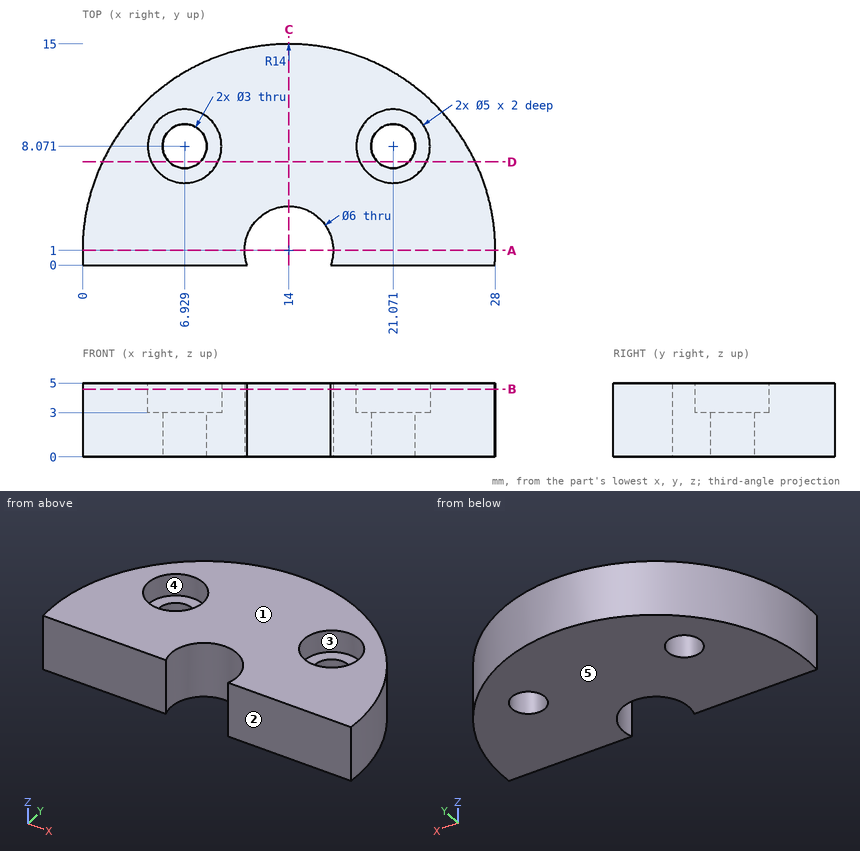
Check sheet for the drawn part. Datum: minimum x, y, z corner. Units: mm. A direction names the side the tool comes from. Round coordinates to 2 decimals unless told otherwise and drop trailing zeros. Loops run counter-clockwise (first coordinate to the right, second up) from the corner with the lowest first, then second, coordinate; pieces in that order, holes last. Notation, with made-up numbers: (-37, 59.25) - (-15, 59.25) arc R28 cw to (-15, 98.25) - close; hole circle Ø3 at (89.5, 28.25). An arc over 180 degrees is marked (long way). Write item = value, one per line. Start each with the question number.
1. Depth check by flat-ended pin: pin 1 (7 mm diameter, centred on x = 14, y = 1, fed in from +Z); pin 2 (1 mm diameter, centred on y = 12, z = 4, fed in from +X); pin 3 (2 mm diameter, centred on x = 13.5, z = 2, fed in from -Y); pin 4 (2 mm diameter, centred on y = 3, z = 4, fed in from -X). Enter the tip coordinate at first touch or a pass-through.
2. Section check C-C on x = 14. Enter the section's corners in (y, z), then the cut area to 3 significant figures.
3. Section check A-A on y = 1. Enter the section's corners in (x, z), then the cut area to 3 significant figures.
4. Mould release check, pull along Y, two halves, no side actions. Record for the marked faces 1, 2 and 3: released by +Y, released by -Y, zero draft, split by the parting line, or undercut.
5. Section check D-D on y = 7. Enter the section's corners in (x, z), then the cut area to 3 significant figures.
6. Section check B-B on z = 4.6. Enter the section's corners in (x, y).
7. Thickness scan on line 1 (X direction, y = 9, z = 4.55); line 2 (X direction, y = 6.25, z = 3.55); line 3 (X direction, y = 1, z = 4). Record the ranges inside material, lowest first.
8. Set-up check for the marked faces 4 and 5: record each of +Z, -Z, +X, -X, +Y, -Y from which the full face is reachable in a straight line by a thin tool's end or side.
Working result:
q1.pin_1 = 5
q1.pin_2 = 23.26
q1.pin_3 = 3.6
q1.pin_4 = 0.04
q2.outline = (4, 0) - (15, 0) - (15, 5) - (4, 5) - close
q2.area = 55.0 mm^2
q3.outline = (0, 0) - (11, 0) - (11, 5) - (0, 5) - close; (17, 0) - (28, 0) - (28, 5) - (17, 5) - close
q3.area = 110 mm^2
q4.face_1 = zero draft
q4.face_2 = released by -Y
q4.face_3 = undercut
q5.outline = (1.35, 0) - (5.88, 0) - (5.88, 3) - (4.67, 3) - (4.67, 5) - (1.35, 5) - close; (7.98, 0) - (20.02, 0) - (20.02, 3) - (18.81, 3) - (18.81, 5) - (9.19, 5) - (9.19, 3) - (7.98, 3) - close; (22.12, 0) - (26.65, 0) - (26.65, 5) - (23.33, 5) - (23.33, 3) - (22.12, 3) - close
q5.area = 95.8 mm^2
q6.outline = (0.04, 0) - (11.17, 0) arc R3 cw (long way) to (16.83, 0) - (27.96, 0) arc R14 ccw (long way) to start; hole circle Ø5 at (6.93, 8.07); hole circle Ø5 at (21.07, 8.07)
q7.line_1 = 2.51 to 4.61, 9.25 to 18.75, 23.39 to 25.49
q7.line_2 = 1.02 to 5.22, 8.64 to 19.36, 22.78 to 26.98
q7.line_3 = 0 to 11, 17 to 28
q8.face_4 = +Z
q8.face_5 = -Z, +X, -X, +Y, -Y
